```python
from build123d import *

# Parameters (mm, degrees)
F0_R     = 4.5
F0_R_2   = 3.6
F1_DEPTH = 30
F0_R_3   = 3
F0_R_4   = 1.75
F2_DEPTH = 3
F3_DEPTH = 2


with BuildPart() as f1:
    # F0 (on Top) → F1 (new body)
    with BuildSketch(Plane.XY):
        Circle(F0_R)
        Circle(F0_R_2, mode=Mode.SUBTRACT)
    extrude(amount=-F1_DEPTH)

    # F0 (on Top) → F2 (join)
    with BuildSketch(Plane.XY):
        Circle(F0_R_2)
        Circle(F0_R_3, mode=Mode.SUBTRACT)
        Circle(F0_R_3)
        Circle(F0_R_4, mode=Mode.SUBTRACT)
    extrude(amount=-F2_DEPTH)

    # F0 (on Top) → F3 (join)
    with BuildSketch(Plane.XY):
        Circle(F0_R_3)
        Circle(F0_R_4, mode=Mode.SUBTRACT)
    extrude(amount=F3_DEPTH)


solid = f1.part
```
Input: part model. Units: mm. Frame: model coordinates. A direction names the side the tool comes from. Round coordinates to 2 decimals unless told otherwise and drop trailing zeros. Order: outer loops, then holes, each group sorted by start corner. A loop starts at its lowest first (then second) coordinate and runs counter-clockwise, first axis right, second up. Notation, with made-up numbers: (82.25, 38) - (126.25, 38) arc R15 cw to (126.25, 43) - close; hole circle Ø5 at (17, -15). An arc over 180 degrees is marked (long way). Answer in a Markdown table with one row per item.
Item 1: Line query: line 1 (Y direction, x = 0, z = 0.65); line 2 (Y direction, x = 0, z = -0.25); line 3 (Z direction, x = 2, y = 3.5). Output: solid intervals per line, ascending.
Model answer:
| item | result |
|---|---|
| line 1 | y = -3 to -1.75, 1.75 to 3 |
| line 2 | y = -4.5 to -1.75, 1.75 to 4.5 |
| line 3 | z = -30 to 0 |
Item 2: Section query A-A (y = 0). Return the cut outline in (x, z), then the cut area to 3 significant figures.
Model answer:
| item | result |
|---|---|
| outline | (-4.5, -30) - (-3.6, -30) - (-3.6, -3) - (-1.75, -3) - (-1.75, 2) - (-3, 2) - (-3, 0) - (-4.5, 0) - close; (1.75, -3) - (3.6, -3) - (3.6, -30) - (4.5, -30) - (4.5, 0) - (3, 0) - (3, 2) - (1.75, 2) - close |
| area | 70.1 mm² |
Item 3: Pin query (flat end, axial travel): pin 1 (2 mm diameter, centred on x = 0.5, y = -1.5, fed in from -Z); pin 2 (4 mm diameter, centred on x = -2.5, y = 1, fed in from -Z); pin 3 (3 mm diameter, centred on x = 2, z = -18.5, fed in from -Y); pin 4 (1 mm diameter, centred on x = 2, z = -5.5, fed in from -Y). Return the tip coordinate at first contact, or that it passes through.
Model answer:
| item | result |
|---|---|
| pin 1 | stops at z = -3 |
| pin 2 | stops at z = -30 |
| pin 3 | stops at y = -4.47 |
| pin 4 | stops at y = -4.24 |
Item 4: Mould query, pull axis X, two halves, no side actions, for faces 4 (the flat face through (1, -3, 0)), 5 (the flat face through (-1, -2, -3)), 6 (the cylindrical face through (-0.59, 4.46, -14.79)). Classes: released by +X, released by -X, zero draft, split by the parting line, or undercut.
Model answer:
| item | result |
|---|---|
| face 4 | zero draft |
| face 5 | undercut |
| face 6 | split by the parting line |
Item 5: Section query C-C (z = -5.5). Return the cut outline in (x, y), then the cut area to 3 significant figures.
Model answer:
| item | result |
|---|---|
| outline | circle Ø9 at (0, 0); hole circle Ø7.2 at (0, 0) |
| area | 22.9 mm² |
Item 6: Reachability of faces 1 (the cylindrical face through (3.434, 1.081, -16.311)), 2 (the flat face through (0, -2, 2)), 3 (the cylindrical face through (-3, 0, 1)) from +Z, -Z, +X, -X, +Y, -Y: full face, straight path, thin tool, end or side. Return the list, or none.
Model answer:
| item | result |
|---|---|
| face 1 | -Z |
| face 2 | +Z, +X, -X, +Y, -Y |
| face 3 | +Z |
